from build123d import *

# Parameters (mm, degrees)
SM_BASE_FLANGE_1_DEPTH = 2325
SKETCH_6_R             = 45
CUT_EXTRUDE_1_DEPTH    = 10
CHAMFER_2_SIZE         = 4


# Sheet-metal steps are written as plain solids
with BuildPart() as part:
    # Sketch 1 → 基体-法兰1 (new body)
    with BuildSketch(Plane.XY):
        with BuildLine():
            Line((0, 0), (43, 0))
            ThreePointArc((43, 0), (52.192388155, -3.807611845), (56, -13))
            Line((56, -13), (56, -137))
            ThreePointArc((56, -137), (52.192388155, -146.192388155), (43, -150))
            Line((43, -150), (0, -150))
            Line((0, -150), (0, -142))
            Line((0, -142), (43, -142))
            ThreePointArc((43, -142), (46.535533906, -140.535533906), (48, -137))
            Line((48, -137), (48, -13))
            ThreePointArc((48, -13), (46.535533906, -9.464466094), (43, -8))
            Line((43, -8), (0, -8))
            Line((0, -8), (0, 0))
        make_face()
    extrude(amount=SM_BASE_FLANGE_1_DEPTH)

    # 草图6 → 切除-拉伸1 (cut)
    with BuildSketch(Plane(origin=(56, 0, 0), x_dir=(0, 0, -1), z_dir=(1, 0, 0))):
        with Locations(Location((-1705, -75, 0), (0, 0, 90))):
            Circle(SKETCH_6_R)
    extrude(amount=-CUT_EXTRUDE_1_DEPTH, mode=Mode.SUBTRACT)

    # 倒角2
    chamfer_2_edges = [part.edges().sort_by_distance(p)[0] for p in [
        (0, 0, 1162.5),
        (0, -150, 1162.5),
    ]]
    chamfer(chamfer_2_edges, length=CHAMFER_2_SIZE)


solid = part.part
Can you work these out from the model? Positions are in its coordinate system, mm. A direction names the side the tool comes from. Coordinates: 2 decimals unless noted, no trailing zeros. Loops run counter-clockwise (first coordinate to the right, second up) from the corner with the lowest first, then second, coordinate; pieces in that order, holes last. Notation, with made-up numbers: (67.25, -8.5) - (120.25, -8.5) arc R14 cw to (120.25, 16.5) - close; hole circle Ø11 at (-35, 83). An arc over 180 degrees is marked (long way). Answer as a JSON object with one key per item and string values. Group by question number.
Item 1: If we mould it in two halves opening along Z, with no side actions, what happens to faces 1 (the face through (56, -74, 1146)), 2 (the face through (49, -69, 2325)), 3 (the face through (49, -69, 0)), 4 (the face through (52.06, -108.17, 1735.41))? For each: released by +Z, released by -Z, zero draft, split by the parting line, or undercut.
Item 2: If we section it at D-D (z = 1408): List the corners of the cut face in (x, y) for me, plus the area to 3 significant figures.
Item 3: If we section it at C-C (z = 1705): List the corners of the cut face in (x, y) for me.
Item 4: If we section it at B-B (y = -75): List the corners of the cut face in (x, z) for me.
Item 5: On a 3-axis mill with a long thin cutter (end or side, diameter ignored), from which of +Z, -Z, +X, -X, +Y, -Y can I reach the whole of each face in a straight line? I mean faces 5 (the face through (23, 0, 1146)), 6 (the face through (21, -142, 1146)). Say none if no direction works.
Item 6: If we section it at A-A (x = 34): List the corners of the cut face in (y, z) for me, plus the area to 3 significant figures.
Item 7: If I drill on L1, parallel to Y at x = 4, z = 841; L2, parallel to Z at x = 52.25, y = -75; L3, parallel to X at y = -124, z = 2084, over which ranges is the centre line in solid material (lowest first)? Write a range as from..to.
Item 8: For pin 1 (8 mm diameter, centred on y = -90.5, z = 1810, fed in from -X), with a flat end and sliding along its axis, tell me the tip position at first contact or that it passes through.
Returned:
{
 "1": {"face 1": "zero draft", "face 2": "released by +Z", "face 3": "released by -Z", "face 4": "undercut"},
 "2": {"outline": "(0, -146) - (4, -150) - (43, -150) arc R13 ccw to (56, -137) - (56, -13) arc R13 ccw to (43, 0) - (4, 0) - (0, -4) - (0, -8) - (43, -8) arc R5 cw to (48, -13) - (48, -137) arc R5 cw to (43, -142) - (0, -142) - close", "area": "1,890 mm²"},
 "3": {"outline": "(0, -146) - (4, -150) - (43, -150) arc R13 ccw to (56, -137) - (56, -120) - (48, -120) - (48, -137) arc R5 cw to (43, -142) - (0, -142) - close; (0, -8) - (43, -8) arc R5 cw to (48, -13) - (48, -30) - (56, -30) - (56, -13) arc R13 ccw to (43, 0) - (4, 0) - (0, -4) - close"},
 "4": {"outline": "(48, 0) - (56, 0) - (56, 1660) - (48, 1660) - close; (48, 1750) - (56, 1750) - (56, 2325) - (48, 2325) - close"},
 "5": {"face 5": "+Z, -Z, +X, -X, +Y", "face 6": "+Z, -Z, -X"},
 "6": {"outline": "(-150, 0) - (-142, 0) - (-142, 2325) - (-150, 2325) - close; (-8, 0) - (0, 0) - (0, 2325) - (-8, 2325) - close", "area": "37,200 mm²"},
 "7": {"L1": "y = -150..-142, -8..0", "L2": "z = 0..1660, 1750..2325", "L3": "x = 48..56"},
 "8": {"pin 1": "stops at x = 48"}
}
